Work out the finished part from the listing and answer in its coordinate system (mm). Face numbers are marked on the shaded views. Give positions to 0.01 mm unless a question says otherwise; leave off trailing zeros. Write each loop counter-clockwise with the first axis right and the second up, starting at its lowest first coordinate (ties: lowest second). Pieces come first, ordered by that corner, then holes.
1) Find section D-D (y = 14.5). Determine the outline of the cut face in (x, z).
2) Find section C-C (x = 16.25). Determine the outline of the cut face in (y, z), plus the area to 3 significant figures.
3) Given pin 1 Ø2 at (x, y) = (9.5, 17.5) entering from +Z; pin 2 Ø5 at (x, z) = (8.5, 9) entering from -Y, each flat-ended and moving along its own axis, determine where each tip first touches the part or whether it passes through.
4) Find section A-A (y = 10). Determine the outline of the cut face in (x, z).
5) Find section B-B (z = 9.25). Determine the outline of the cut face in (x, y), plus the area to 3 significant figures.
6) Straight lines are drawn through the part: probe 1 along Y at (x, z) = (12.5, 3.5); probe 2 along X at (y, z) = (9.75, 9.5); probe 3 along Y at (x, z) = (11.5, 4). For each, find the intervals that lie inside material, in ascending order.
7) Determine the mould class of the marked faces 1, 2 and 3 for opening direction Y: pulls with the +Y half, pulls with the -Y half, needs draft (parallel to the pull), parting line crosses it, or undercut.
```python
from build123d import *

# Parameters (mm, degrees)
BOSS_EXTRU_1_DEPTH      = 10
CONG_1_R                = 5
ESQUISSE2_R             = 1.5
ENL_V_MAT_EXTRU_1_DEPTH = 10


with BuildPart() as part:
    # Esquisse1 → Boss.-Extru.1 (new body)
    with BuildSketch(Plane.XY):
        with BuildLine():
            Line((5, 0), (20, 0))
            Line((20, 0), (20, 20))
            Line((20, 20), (5, 20))
            ThreePointArc((5, 20), (1.464466094, 18.535533906), (0, 15))
            Line((0, 15), (0, 5))
            ThreePointArc((0, 5), (1.464466094, 1.464466094), (5, 0))
        make_face()
    extrude(amount=BOSS_EXTRU_1_DEPTH)

    # Congé1
    cong_1_edges = [part.edges().sort_by_distance(p)[0] for p in [
        (1.464466094, 18.535533906, 10),
        (0, 10, 10),
        (1.464466094, 1.464466094, 10),
        (12.5, 0, 10),
        (12.5, 20, 10),
    ]]
    fillet(cong_1_edges, radius=CONG_1_R)

    # Esquisse2 → Enlèv. mat.-Extru.1 (cut)
    with BuildSketch(Plane.XY.offset(10)):
        with Locations((12.5, 10)):
            Circle(ESQUISSE2_R)
    extrude(amount=-ENL_V_MAT_EXTRU_1_DEPTH, mode=Mode.SUBTRACT)


solid = part.part
```
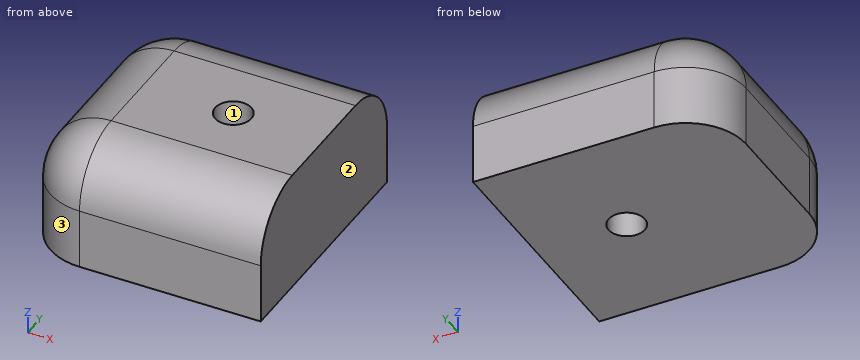
Results:
1. outline: (0, 0) - (20, 0) - (20, 10) - (5, 10) arc R5 ccw to (0, 5) - close
2. outline: (0, 0) - (20, 0) - (20, 5) arc R5 ccw to (15, 10) - (5, 10) arc R5 ccw to (0, 5) - close
2. area: 189 mm2
3. pin 1: stops at z = 9.77
3. pin 2: stops at y = 0.23
4. outline: (0, 0) - (11, 0) - (11, 10) - (5, 10) arc R5 ccw to (0, 5) - close; (14, 0) - (20, 0) - (20, 10) - (14, 10) - close
5. outline: (2.37, 5) arc R2.63 ccw to (5, 2.37) - (20, 2.37) - (20, 17.63) - (5, 17.63) arc R2.63 ccw to (2.37, 15) - close; hole circle Ø3 at (12.5, 10)
5. area: 259 mm2
6. probe 1: y = 0 to 8.5, 11.5 to 20
6. probe 2: x = 2.82 to 11.02, 13.98 to 20
6. probe 3: y = 0 to 8.88, 11.12 to 20
7. face 1: undercut
7. face 2: needs draft
7. face 3: pulls with the -Y half
